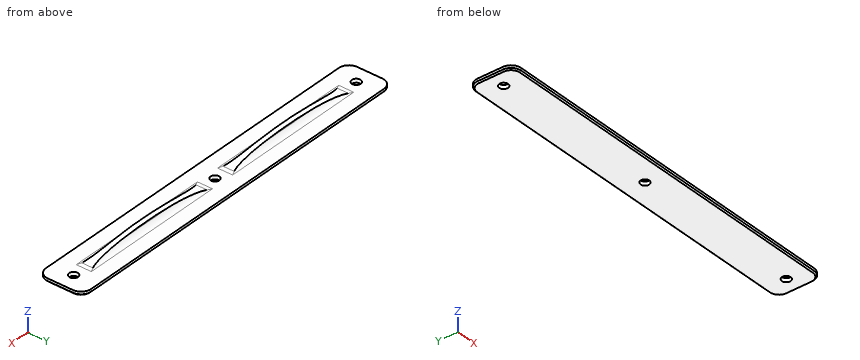
Autodesk Inventor part; units mm, degrees
ref_plane "YZ Plane" through (0, 0, 0) normal (1, 0, 0) x (0, 1, 0)
ref_plane "XZ Plane" through (0, 0, 0) normal (0, 1, 0) x (-1, 0, 0)
ref_plane "XY Plane" through (0, 0, 0) normal (0, 0, 1) x (1, 0, 0)
sketch "Sketch1" plane through (0, 0, 0) normal (0, 0, 1) x (1, 0, 0)
  line L0 (71, -9) -> (-71, -9)
  line L1 (-75, -5) -> (-75, 5)
  line L2 (-71, 9) -> (71, 9)
  line L3 (75, 5) -> (75, -5)
  line L4 (75, -9) -> (-75, 9) construction
  line L5 (-75, -9) -> (75, 9) construction
  arc A0 (-71, 9) -> (-75, 5) centre (-71, 5) ccw
  arc A1 (-75, -5) -> (-71, -9) centre (-71, -5) ccw
  arc A2 (75, 5) -> (71, 9) centre (71, 5) ccw
  arc A3 (71, -9) -> (75, -5) centre (71, -5) ccw
  circle A4 centre (0, 0) radius 1.75
  line L6 (-75, 0) -> (-68.5, 0) construction
  line L7 (75, 0) -> (68.5, 0) construction
  circle A5 centre (-68.5, 0) radius 1.75
  circle A6 centre (68.5, 0) radius 1.75
  dimension "d0" = 4
  dimension "d2" = 150
  dimension "d3" = 18
  dimension "d4" = 3.5
  dimension "d5" = 6.5
  dimension "d6" = 6.5
extrude "Extrusion1" add sketch "Sketch1" along normal blind 1.5
sketch "Sketch2" plane through (0, 0, 0) normal (0, 1, 0) x (-1, 0, 0)
  line L0 (71, 1.5) -> (-71, 1.5)
  arc A0 (62.75, 1.5) -> (5.75, 1.5) centre (34.25, -159.7) ccw
  line L1 (-1.75, 1.5) -> (1.75, 1.5)
  line L2 (0, 1.5) -> (0, 8.4786) construction
  line L3 (66.75, 1.5) -> (70.25, 1.5)
  line L4 (66.75, 1.5) -> (62.75, 1.5) construction
  line L5 (5.75, 1.5) -> (1.75, 1.5) construction
  line L6 (1.75, 1.5) -> (1.75, 0)
  line L7 (46.1417, 4) -> (24.4242, 4) construction
  point P0 (0, 0)
  dimension "d9" = 4
  dimension "d10" = 2.5
extrude "Extrusion2" add sketch "Sketch2" along normal mid plane 2
fillet "Fillet1" radius 2 2 edges at (-34.25, -1, 1.5) (-34.25, 1, 1.5)
fillet "Fillet1" radius 10 2 edges at (-62.75, 0, 1.5) (-5.75, 0, 1.5)
mirror "Mirror1" about plane through (0, 0, 0) normal (1, 0, 0) of "Extrusion2", "Fillet1"
chamfer "Chamfer1" distance 0.5 angle 45 8 edges at (0, -9, 0) (73.8284, -7.8284, 0) (75, 0, 0) (73.8284, 7.8284, 0) (0, 9, 0) (-73.8284, 7.8284, 0) (-75, 0, 0) (-73.8284, -7.8284, 0)
properties part number "LEDLid"
Verification items for the finished model (mm, model axes). Give positions to 0.01 mm unless a question says otherwise; leave off trailing zeros. Order: outer loops, then holes, each group sorted by start corner. A loop starts at its lowest first (then second) coordinate and runs counter-clockwise, first axis right, second up. Notation, with made-up numbers: (11, -11.75) -> (28, -11.75) arc R22 cw to (28, 0.25) -> close; hole circle Ø9 at (23, 78). An arc over 180 degrees is marked (long way). Answer as CSV lines item,"result".
Q1. Sectioned sample at A-A on x = 0. Record the cut outline in (y, z).
Solutions:
outline,"(-9, 0.5) -> (-8.5, 0) -> (-1.75, 0) -> (-1.75, 1.5) -> (-9, 1.5) -> close; (1.75, 0) -> (8.5, 0) -> (9, 0.5) -> (9, 1.5) -> (1.75, 1.5) -> close"
Q2. Sectioned sample at C-C on x = -31. Record the cut outline in (y, z), plus the area to 3 significant figures.
Solutions:
outline,"(-9, 0.5) -> (-8.5, 0) -> (8.5, 0) -> (9, 0.5) -> (9, 1.5) -> (3, 1.5) arc R2 cw to (1, 3.5) -> (1, 3.97) -> (-1, 3.97) -> (-1, 3.5) arc R2 cw to (-3, 1.5) -> (-9, 1.5) -> close"
area,"33.4 mm²"
Q3. Sectioned sample at D-D on x = 57. Record the cut outline in (y, z), plus the area to 3 significant figures.
Solutions:
outline,"(-9, 0.5) -> (-8.5, 0) -> (8.5, 0) -> (9, 0.5) -> (9, 1.5) -> (3, 1.5) arc R2 cw to (1.32, 2.41) -> (-1.32, 2.41) arc R2 cw to (-3, 1.5) -> (-9, 1.5) -> close"
area,"30.1 mm²"
Q4. Sectioned sample at B-B on z = 2.85. Record the cut outline in (x, y).
Solutions:
outline,"(-53.62, -1.11) -> (-14.88, -1.11) -> (-14.88, 1.11) -> (-53.62, 1.11) -> close; (14.88, -1.11) -> (53.62, -1.11) -> (53.62, 1.11) -> (14.88, 1.11) -> close"
Q5. Depth check by flat-ended pin: pin 1 (5 mm diameter, centred on x = -27, y = 7, fed in from +Z); pin 2 (3 mm diameter, centred on x = -68.5, y = 0, fed in from -Z); pin 3 (8 mm diameter, centred on x = -58, y = -1.5, fed in from +Z); pin 4 (0.6 mm diameter, centred on x = -40.5, z = 4, fed in from +Y). Enter the tip coordinate at first touch or a pass-through.
Solutions:
pin 1,"stops at z = 1.5"
pin 2,"passes through"
pin 3,"stops at z = 2.8"
pin 4,"stops at y = 1"
Q6. Scan lines: probe 1 along Y at (x, z) = (0, 0.6); probe 2 along X at (y, z) = (0.5, 0.3); probe 3 along Z at (x, y) = (-3.5, -5). Record each from-to range of solid material in increasing order.
Solutions:
probe 1,"y = -9 to -1.75, 1.75 to 9"
probe 2,"x = -74.8 to -70.18, -66.82 to -1.68, 1.68 to 66.82, 70.18 to 74.8"
probe 3,"z = 0 to 1.5"
